from build123d import *

# Parameters (mm, degrees)
F2_R     = 15.75
F0_R     = 26.5
F4_DEPTH = 25
F5_DEPTH = 25


with BuildPart() as f3:
    # F2 (on offset) → F3 section 0
    with BuildSketch(Plane.XY.offset(25)):
        Circle(F2_R)
    # F0 (on Top) → F3 section 1
    with BuildSketch(Plane.XY):
        Circle(F0_R)
    loft()

    # F4 (add): a face of the model
    f4_faces = [f3.faces().sort_by_distance(p)[0] for p in [
        (0, 0, 25),
    ]]
    extrude(f4_faces, amount=F4_DEPTH)

    # F5 (add): a face of the model
    f5_faces = [f3.faces().sort_by_distance(p)[0] for p in [
        (0, 0, 0),
    ]]
    extrude(f5_faces, amount=F5_DEPTH)


solid = f3.part
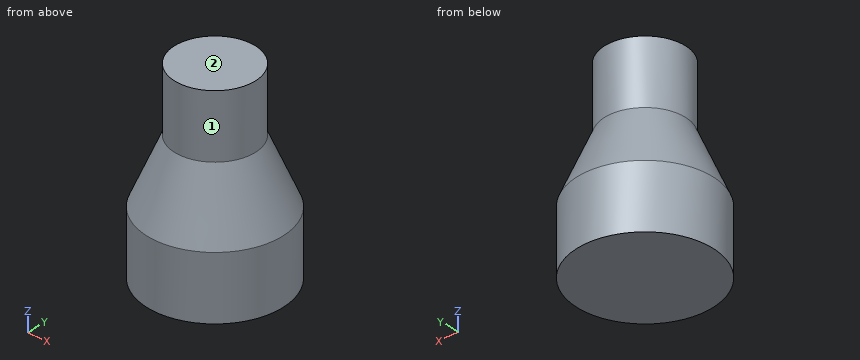
Geometry check sheet. Reference: the model listing, model coordinates, mm. Face numbers are marked on the shaded views. A direction names the side the tool comes from. Coordinates: 2 decimals unless noted, no trailing zeros. Loops run counter-clockwise (first coordinate to the right, second up) from the corner with the lowest first, then second, coordinate; pieces in that order, holes last. Notation, with made-up numbers: (-16.75, 51.25) - (30.25, 51.25) arc R18 ccw to (30.25, 80.25) - close; hole circle Ø7 at (27, 4). An arc over 180 degrees is marked (long way). Use one line per item in the form item = value. Start each with the question number.
Item 1: Section check A-A, the plane x = 0. Enter the section's corners in (y, z).
Item 2: Gauge pin test, flat ends, axial feed: pin 1 (1.5 mm diameter, centred on y = 18, z = 7.5, fed in from +X); pin 2 (1 mm diameter, centred on x = 9.5, z = -5.5, fed in from -Y); pin 3 (2 mm diameter, centred on y = 9, z = 0.5, fed in from -X). Record the tip position at first contact, or that the pin passes through.
Item 3: Thickness scan on probe 1 along Y at (x, z) = (10, -16); probe 2 along Y at (x, z) = (-22.5, 1); probe 3 along X at (y, z) = (-12, 34). Record the ranges inside material, lowest first.
Item 4: Section check C-C, the plane z = 6. Enter the section's corners in (x, y), and give its area (3 significant figures).
Item 5: Tool access check on the marked faces 1 and 2. Record the directions out of +Z, -Z, +X, -X, +Y, -Y that give a thin tool (end or side, any length) a straight path to the whole face; none if there is none.
Item 6: Section check B-B, the plane z = 16. Enter the section's corners in (x, y), and give its area (3 significant figures).
Computed:
q1.outline = (-26.5, -25) - (26.5, -25) - (26.5, 0) - (15.75, 25) - (15.75, 50) - (-15.75, 50) - (-15.75, 25) - (-26.5, 0) - close
q2.pin_1 = 15.75
q2.pin_2 = -24.92
q2.pin_3 = -25.22
q3.probe_1 = -24.54 to 24.54
q3.probe_2 = -13.17 to 13.17
q3.probe_3 = -10.2 to 10.2
q4.outline = circle Ø47.84 at (0, 0)
q4.area = 1,800 mm2
q5.face_1 = +Z
q5.face_2 = +Z, +X, -X, +Y, -Y
q6.outline = circle Ø39.24 at (0, 0)
q6.area = 1,210 mm2
